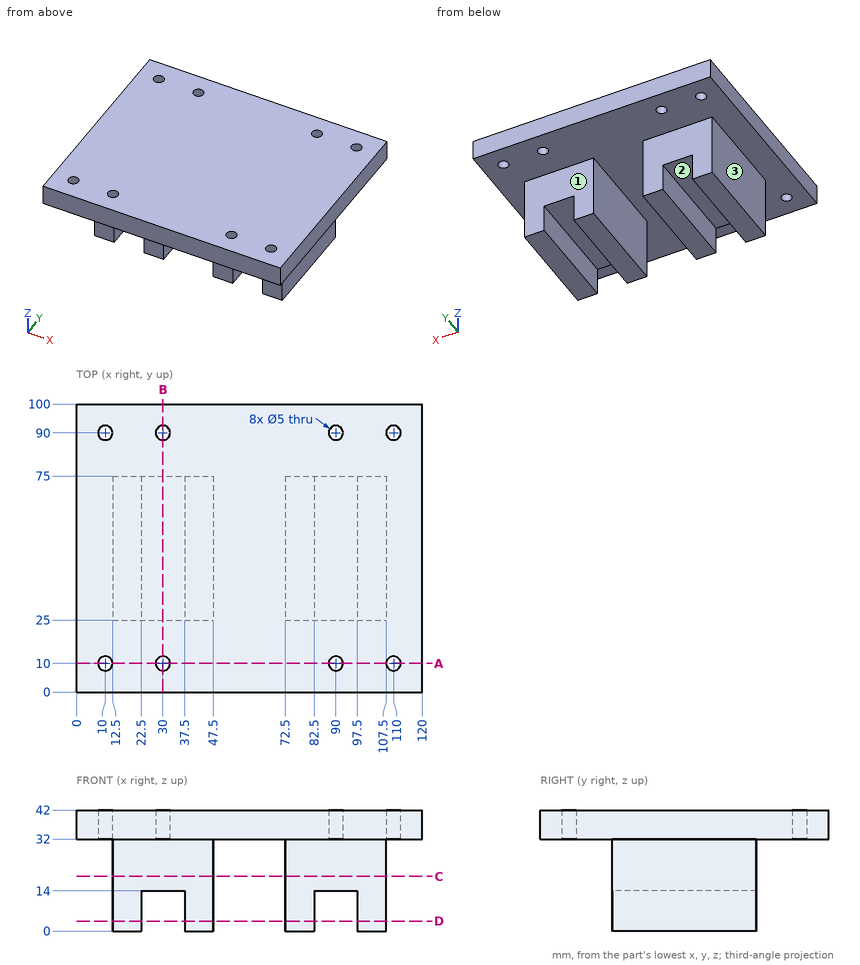
Could you check a few things on this drawing? It's one solid part, dimensions in mm from its lowest x, y, z. A direction names the side the tool comes from. Coordinates: 2 decimals unless noted, no trailing zeros. Order: outer loops, then holes, each group sorted by start corner. A loop starts at its lowest first (then second) coordinate and runs counter-clockwise, first axis right, second up. Notation, with made-up numbers: M -17.75,3 L -9.75,3 A31 ccw -9.75,35 Z; hole C 8,63 d4. An arc over 180 degrees is marked long. Use a Markdown table: item, result. Add a question column.
Q1. If I drill on L1, parallel to X at y = 58.5, z = 13; L2, parallel to Y at x = 90, z = 37; L3, parallel to X at y = 50.5, z = 28, over which ranges is the centre line in solid material (lowest first)?
Q2. I want a section at C-C on z = 19. List the corners of the cut face in (x, y) for me.
Q3. I want a section at A-A on y = 10. List the corners of the cut face in (x, z) for me, then the cut area to 3 significant figures.
Q4. Which directions (+Z, -Z, +X, -X, +Y, -Y) give clear straight access to the entire face, cutting with the end or side of a thin tool? Please do the marked faces 1, 2 and 3.
Q5. I want a section at D-D on z = 3.5. List the corners of the cut face in (x, y) for me, then the cut area to 3 significant figures.
Q6. I want a section at B-B on x = 30. List the corners of the cut face in (y, z) for me.
Q7. I'm going to push flat-ended pins straight in: pin 1 (4.5 mm diameter, centred on x = 90.5, y = 55.5, fed in from -Z); pin 2 (9.5 mm diameter, centred on y = 59.5, z = 22, fed in from -X); pin 3 (6 mm diameter, centred on x = 92, z = 25, fed in from +Y). Where does each tip first touch, or does it pass through?
Checked values:
| question | item | result |
|---|---|---|
| 1 | L1 | 12.5 to 22.5, 37.5 to 47.5, 72.5 to 82.5, 97.5 to 107.5 |
| 1 | L2 | 0 to 7.5, 12.5 to 87.5, 92.5 to 100 |
| 1 | L3 | 12.5 to 47.5, 72.5 to 107.5 |
| 2 | outline | M 12.5,25 L 47.5,25 L 47.5,75 L 12.5,75 Z; M 72.5,25 L 107.5,25 L 107.5,75 L 72.5,75 Z |
| 3 | outline | M 0,32 L 7.5,32 L 7.5,42 L 0,42 Z; M 12.5,32 L 27.5,32 L 27.5,42 L 12.5,42 Z; M 32.5,32 L 87.5,32 L 87.5,42 L 32.5,42 Z; M 92.5,32 L 107.5,32 L 107.5,42 L 92.5,42 Z; M 112.5,32 L 120,32 L 120,42 L 112.5,42 Z |
| 3 | area | 1,000 mm² |
| 4 | face 1 | -Z, +X, -X, +Y |
| 4 | face 2 | -Z, +Y, -Y |
| 4 | face 3 | -Z, -X, +Y, -Y |
| 5 | outline | M 12.5,25 L 22.5,25 L 22.5,75 L 12.5,75 Z; M 37.5,25 L 47.5,25 L 47.5,75 L 37.5,75 Z; M 72.5,25 L 82.5,25 L 82.5,75 L 72.5,75 Z; M 97.5,25 L 107.5,25 L 107.5,75 L 97.5,75 Z |
| 5 | area | 2,000 mm² |
| 6 | outline | M 0,32 L 7.5,32 L 7.5,42 L 0,42 Z; M 12.5,32 L 25,32 L 25,14 L 75,14 L 75,32 L 87.5,32 L 87.5,42 L 12.5,42 Z; M 92.5,32 L 100,32 L 100,42 L 92.5,42 Z |
| 7 | pin 1 | z = 14 |
| 7 | pin 2 | x = 12.5 |
| 7 | pin 3 | y = 75 |
